from build123d import *

# Parameters (mm, degrees)
BOSS_EXTRUDE1_DEPTH       = 47.9
F_3_0MM_DOWEL_HOLE1_D     = 3
F_3_0MM_DOWEL_HOLE1_DEPTH = 8.5
F_3_0MM_DOWEL_HOLE1_TIP   = 0.901290929


with BuildPart() as part:
    # Sketch1 → Boss-Extrude1 (new body, symmetric)
    with BuildSketch(Plane(origin=(0, 0, 0), x_dir=(0, 0, -1), z_dir=(1, 0, 0))):
        Polygon((-8.5, 0), (8.5, 0), (8.5, 5), (5.1, 5), (5.1, 2), (-5.1, 2), (-5.1, 5), (-8.5, 5), align=None)
    extrude(amount=BOSS_EXTRUDE1_DEPTH, both=True)

    # Ø3.0mm Dowel Hole1
    with Locations(Plane(origin=(0, 2, 0), x_dir=(1, 0, 0), z_dir=(0, 1, 0))):
        with Locations((-30.875, 0), (30.875, 0)):
            Hole(F_3_0MM_DOWEL_HOLE1_D / 2, depth=F_3_0MM_DOWEL_HOLE1_DEPTH)
            with Locations((0, 0, -(F_3_0MM_DOWEL_HOLE1_DEPTH + F_3_0MM_DOWEL_HOLE1_TIP / 2))):  # 118° drill point
                Cone(0, F_3_0MM_DOWEL_HOLE1_D / 2, F_3_0MM_DOWEL_HOLE1_TIP, mode=Mode.SUBTRACT)


solid = part.part
Check sheet for the modelled part. Datum: model origin and axes. Units: mm. A direction names the side the tool comes from. Round coordinates to 2 decimals unless told otherwise and drop trailing zeros. Order: outer loops, then holes, each group sorted by start corner. A loop starts at its lowest first (then second) coordinate and runs counter-clockwise, first axis right, second up. Notation, with made-up numbers: M -13.5,10 L 18.5,10 A20 ccw 18.5,49 Z; hole C 28,46.25 d8. An arc over 180 degrees is marked long. One line per item, written item: value. Start each with the question number.
1. Gauge pin test, flat end, axial feed: P1, Ø2, axis at x = 0.5, z = -2.5, coming from the +Y side. Record the tip position at first contact, or that the pin passes through.
2. Access from +Z, -Z, +X, -X, +Y, -Y to the whole of each face (thin tool, end or side, straight path). Record for faces 4 (the flat face through (1, 4, -5.1)), 5 (the flat face through (47.9, 1, 0)).
3. Release check for a two-part mould opening along Z. For faces 1 (the flat face through (1, 3, 8.5)), 2 (the flat face through (1, 3, 5.1)), 3 (the flat face through (1, 0, 0)) record: released by +Z, released by -Z, zero draft, split by the parting line, or undercut.
4. Section check D-D on z = 3.75. Enter the section's corners in (x, y), and give its area (3 significant figures).
5. Scan lines: line 1 along Z through (x, y) = (16, 4.8); line 2 along Y through (x, z) = (-3, 4.25). Record each from-to range of solid material in increasing order.
6. Section check A-A on z = 0. Enter the section's corners in (x, y) (3 decimals).
7. Section check B-B on y = 3.5. Enter the section's corners in (x, z), and give its area (3 significant figures).
8. Section check C-C on x = -7.5. Enter the section's corners in (y, z), and give its area (3 significant figures).
Results found:
1. P1: y = 2
2. face 4: +X, -X, +Y
2. face 5: +Z, -Z, +X, +Y, -Y
3. face 1: released by +Z
3. face 2: undercut
3. face 3: zero draft
4. outline: M -47.9,0 L 47.9,0 L 47.9,2 L -47.9,2 Z
4. area: 192 mm^2
5. line 1: -8.5 to -5.1, 5.1 to 8.5
5. line 2: 0 to 2
6. outline: M -47.9,0 L -32.375,0 L -32.375,2 L -47.9,2 Z; M -29.375,0 L 29.375,0 L 29.375,2 L -29.375,2 Z; M 32.375,0 L 47.9,0 L 47.9,2 L 32.375,2 Z
7. outline: M -47.9,-8.5 L 47.9,-8.5 L 47.9,-5.1 L -47.9,-5.1 Z; M -47.9,5.1 L 47.9,5.1 L 47.9,8.5 L -47.9,8.5 Z
7. area: 651 mm^2
8. outline: M 0,-8.5 L 5,-8.5 L 5,-5.1 L 2,-5.1 L 2,5.1 L 5,5.1 L 5,8.5 L 0,8.5 Z
8. area: 54.4 mm^2
